```python
from build123d import *

# Parameters (mm, degrees)
SKETCH2_W             = 127
SKETCH2_H             = 152.4
BOSS_EXTRUDE2_DEPTH   = 6.35
SKETCH3_W             = 127
SKETCH3_H             = 65.278
CUT_EXTRUDE1_DEPTH    = 100.3932216
CAVITY1_START         = -63.5
CAVITY1_OUTLINE_W     = 28.919714286
CAVITY1_OUTLINE_H     = 6.35
CAVITY1_OUTLINE_W_2   = 29.028571429
CAVITY1_DEPTH         = 6.35
CAVITY1_START_2       = 57.15
CAVITY1_2_OUTLINE_W   = 28.919714286
CAVITY1_2_OUTLINE_H   = 6.35
CAVITY1_2_OUTLINE_W_2 = 29.028571429
CAVITY1_2_DEPTH       = 6.35
CUT_EXTRUDE2_DEPTH    = 100.3932216
BOSS_EXTRUDE3_DEPTH   = 6.35
CAVITY2_START         = 17.018
CAVITY2_OUTLINE_W     = 20.9
CAVITY2_OUTLINE_H     = 9
CAVITY2_OUTLINE_W_2   = 25.4
CAVITY2_OUTLINE_W_3   = 19.05
CAVITY2_DEPTH         = 6.35
SKETCH6_W             = 6.35
SKETCH6_H             = 6.059714286
BOSS_EXTRUDE4_DEPTH   = 6.35
SKETCH7_W             = 114.3
SKETCH7_H             = 29.173714286
CUT_EXTRUDE3_DEPTH    = 100.658360693


# Read off the part's stored shape, not the designer's step: Cavity1, Cavity2
with BuildPart() as part:
    # Sketch2 → Boss-Extrude2 (new body)
    with BuildSketch(Plane.XY):
        Rectangle(SKETCH2_W, SKETCH2_H)
    extrude(amount=BOSS_EXTRUDE2_DEPTH)

    # Sketch3 → Cut-Extrude1 (cut, through all)
    with BuildSketch(Plane.XY.offset(6.35)):
        with Locations((0, 43.561)):
            Rectangle(SKETCH3_W, SKETCH3_H)
    extrude(amount=-CUT_EXTRUDE1_DEPTH, mode=Mode.SUBTRACT)

    # Cavity1 outline → Cavity1 (cut)
    with BuildSketch(Plane.YZ.offset(CAVITY1_START)):
        with Locations((-3.537857143, 3.175)):
            Rectangle(CAVITY1_OUTLINE_W, CAVITY1_OUTLINE_H)
        with Locations((-61.540571429, 3.175)):
            Rectangle(CAVITY1_OUTLINE_W_2, CAVITY1_OUTLINE_H)
    extrude(amount=CAVITY1_DEPTH, mode=Mode.SUBTRACT)

    # Cavity1 2 outline → Cavity1 2 (cut)
    with BuildSketch(Plane.YZ.offset(CAVITY1_START_2)):
        with Locations((-3.537857143, 3.175)):
            Rectangle(CAVITY1_2_OUTLINE_W, CAVITY1_2_OUTLINE_H)
        with Locations((-61.540571429, 3.175)):
            Rectangle(CAVITY1_2_OUTLINE_W_2, CAVITY1_2_OUTLINE_H)
    extrude(amount=CAVITY1_2_DEPTH, mode=Mode.SUBTRACT)

    # Sketch4 → Cut-Extrude2 (cut, through all)
    with BuildSketch(Plane(origin=(0, 0, 0), x_dir=(-1, 0, 0), z_dir=(0, 0, -1))):
        Polygon((-57.15, -76.054857143), (-57.15, -79.645008966), (-65.377811093, -79.645008966), (-65.377811093, -73.782579567), (-57.15, -73.782579567), align=None)
        Polygon((57.15, -76.054857143), (57.15, -79.645008966), (65.72742819, -79.645008966), (65.72742819, -72.849920344), (57.15, -72.849920344), align=None)
    extrude(amount=-CUT_EXTRUDE2_DEPTH, mode=Mode.SUBTRACT)

    # Sketch5 → Boss-Extrude3 (add, through all)
    with BuildSketch(Plane(origin=(0, 0, 0), x_dir=(-1, 0, 0), z_dir=(0, 0, -1))):
        Polygon((-57.15, 10.922), (-57.15, 23.368), (57.995680603, 23.368), (57.15, 10.922), align=None)
    extrude(amount=-BOSS_EXTRUDE3_DEPTH)

    # Cavity2 outline → Cavity2 (cut)
    with BuildSketch(Plane(origin=(0, 0, 0), x_dir=(1, 0, 0), z_dir=(0, 1, 0)).offset(CAVITY2_START)):
        with Locations((-48.55, -3.5)):
            Rectangle(CAVITY2_OUTLINE_W, CAVITY2_OUTLINE_H)
        with Locations((0, -3.5)):
            Rectangle(CAVITY2_OUTLINE_W_2, CAVITY2_OUTLINE_H)
        with Locations((47.625, -3.5)):
            Rectangle(CAVITY2_OUTLINE_W_3, CAVITY2_OUTLINE_H)
    extrude(amount=CAVITY2_DEPTH, mode=Mode.SUBTRACT)

    # Sketch6 → Boss-Extrude4 (add, through all)
    with BuildSketch(Plane.XY.offset(6.35)):
        with Locations((60.325, 13.988142857)):
            Rectangle(SKETCH6_W, SKETCH6_H)
        Polygon((-63.914210908, 17.018), (-57.564210908, 17.018), (-57.15, 10.922), (-63.914210908, 10.922), align=None)
    extrude(amount=-BOSS_EXTRUDE4_DEPTH)

    # Sketch7 → Cut-Extrude3 (cut, through all)
    with BuildSketch(Plane(origin=(0, 0, 0), x_dir=(-1, 0, 0), z_dir=(0, 0, -1))):
        with Locations((0, -61.613142857)):
            Rectangle(SKETCH7_W, SKETCH7_H)
    extrude(amount=-CUT_EXTRUDE3_DEPTH, mode=Mode.SUBTRACT)


solid = part.part
```
The model under review builds one solid part; all positions refer to its coordinate system, in mm. A direction names the side the tool comes from. Round coordinates to 2 decimals unless told otherwise and drop trailing zeros. Write each loop counter-clockwise with the first axis right and the second up, starting at its lowest first coordinate (ties: lowest second). Pieces come first, ordered by that corner, then holes. Notation, with made-up numbers: (57.25, 76) - (90.25, 76) arc R22 cw to (90.25, 106) - close; hole circle Ø6 at (18.25, 81.5). An arc over 180 degrees is marked (long way). One line per question, with ' | ' between items.
Item 1: The part is to be moulded in two halves that separate along Y. For faces 5 (the face through (26, 23.368, 3)), 6 (the face through (-1, -11, 6.35)), 7 (the face through (57.15, -4, 3)), say which applies: pulls with the +Y half, pulls with the -Y half, needs draft (parallel to the pull), parting line crosses it, or undercut.
Resolved:
face 5: pulls with the +Y half | face 6: needs draft | face 7: undercut
Item 2: For P1, Ø3, axis at y = 21, z = 3.5, coming from the +X side; P2, Ø3, axis at x = -55, z = 4.5, coming from the +Y side; P3, Ø3, axis at y = -2, z = 4, coming from the +X side, all flat-tipped, find the tip position at first contact; note any pin that passes through.
Resolved:
P1: stops at x = 38.1 | P2: stops at y = 17.02 | P3: stops at x = 57.15
Item 3: Add section B-B, the plane x = 49.5. Give the boundary of the cut face in (y, z).
Resolved:
outline: (-47.03, 0) - (17.02, 0) - (17.02, 6.35) - (-47.03, 6.35) - close
Item 4: Add section C-C, the plane y = -13.5. Give the boundary of the cut face in (x, z), then the cut area to 3 significant figures.
Resolved:
outline: (-57.15, 0) - (57.15, 0) - (57.15, 6.35) - (-57.15, 6.35) - close | area: 726 mm2
Item 5: For faces 1 (the face through (38.1, 20, 3)), 2 (the face through (-12.7, 20, 3)), 3 (the face through (60, -17.998, 3)), 4 (the face through (-60, -17.998, 3)), list the 3-axis set-ups (+Z, -Z, +X, -X, +Y, -Y) from which the entire face can be reached by the end or side of a thin tool; tool diameter is ignored.
Resolved:
face 1: +Z, -Z, +X, +Y | face 2: +Z, -Z, +Y | face 3: +Z, -Z, +X | face 4: +Z, -Z, -X
Item 6: Add section A-A, the plane z = 1. Give the boundary of the cut face in (x, y), then the cut area to 3 significant figures.
Resolved:
outline: (-63.91, 10.92) - (-57.15, 10.92) - (-57.15, -18) - (-63.5, -18) - (-63.5, -47.03) - (63.5, -47.03) - (63.5, -18) - (57.15, -18) - (57.15, 10.96) - (63.5, 10.96) - (63.5, 17.02) - (38.1, 17.02) - (38.1, 23.37) - (12.7, 23.37) - (12.7, 17.02) - (-12.7, 17.02) - (-12.7, 23.37) - (-38.1, 23.37) - (-38.1, 17.02) - (-63.91, 17.02) - close | area: 8,090 mm2
Item 7: To check wall thickness, follow probe 1 along Y at (x, z) = (-58, 1); probe 2 along X at (y, z) = (-8, 5); probe 3 along X at (y, z) = (-25, 3.25). State the ranges of each line that lie inside material, in increasing order.
Resolved:
probe 1: y = -47.03 to -18, 10.92 to 17.02 | probe 2: x = -57.15 to 57.15 | probe 3: x = -63.5 to 63.5
